from build123d import *

# Parameters (mm, degrees)
F0_W     = 3
F0_H     = 20
F0_W_2   = 2
F0_H_2   = 4
F1_DEPTH = 3
F3_W     = 4
F3_H     = 2
F4_DEPTH = 3


with BuildPart() as f1:
    # F0 (on Top) → F1 (new body)
    with BuildSketch(Plane.XY):
        Polygon((-25, 0), (-30, 0), (-30, -50), (0, 0), align=None)
        with Locations((-23.5, -20)):
            Rectangle(F0_W, F0_H, mode=Mode.SUBTRACT)
        Polygon((0, 0), (-30, -50), (-30, -100), (0, -100), (30, -100), (30, -50), (30, 0), align=None)
        with Locations((-23.5, -80)):
            Rectangle(F0_W, F0_H, mode=Mode.SUBTRACT)
        Polygon((12.9807621135, -87.5470053838), (0, -80.0525588833), (-0.0096189432, -80.0470053838), (-13, -87.5470053838), (-13, -81.7735026919), (-0.0096189432, -74.2735026919), (12.9807621135, -81.7735026919), align=None, mode=Mode.SUBTRACT)
        Polygon((-13, -70), (-0.0096189432, -62.5), (12.9807621135, -70), (12.9807621135, -75.7735026919), (-0.0096189432, -68.2735026919), (-13, -75.7735026919), align=None, mode=Mode.SUBTRACT)
        with Locations((23.5, -80)):
            Rectangle(F0_W, F0_H, mode=Mode.SUBTRACT)
        with Locations((28, -52)):
            Rectangle(F0_W_2, F0_H_2, mode=Mode.SUBTRACT)
        Polygon((-12.9903810568, -39.2735026919), (0, -31.7735026919), (12.9903810568, -39.2735026919), (12.9903810568, -45.0470053838), (0, -37.5470053838), (-12.9903810568, -45.0470053838), align=None, mode=Mode.SUBTRACT)
        Polygon((-12.9903810568, -27.5), (0, -20), (12.9903810568, -27.5), (12.9903810568, -33.2735026919), (0, -25.7735026919), (-12.9903810568, -33.2735026919), align=None, mode=Mode.SUBTRACT)
        with Locations((23.5, -20)):
            Rectangle(F0_W, F0_H, mode=Mode.SUBTRACT)
    extrude(amount=F1_DEPTH)

    # F3 (on offset) → F4 (cut, through all)
    with BuildSketch(Plane.YZ.offset(30)):
        with Locations((-52, 1.5)):
            Rectangle(F3_W, F3_H)
    extrude(amount=-F4_DEPTH, mode=Mode.SUBTRACT)


solid = f1.part
Check sheet for the modelled part. Datum: model origin and axes. Units: mm. Coordinates: 2 decimals unless noted, no trailing zeros. Write each loop counter-clockwise with the first axis right and the second up, starting at its lowest first coordinate (ties: lowest second). Pieces come first, ordered by that corner, then holes.
Item 1: Cross-section at A-A on y = -89. Record the boundary of the cut face in (x, z), then the cut area to 3 significant figures.
Numbers:
outline: (-30, 0) - (-25, 0) - (-25, 3) - (-30, 3) - close; (-22, 0) - (22, 0) - (22, 3) - (-22, 3) - close; (25, 0) - (30, 0) - (30, 3) - (25, 3) - close
area: 162 mm2
Item 2: Cross-section at D-D on y = -36.5. Record the boundary of the cut face in (x, z), then the cut area to 3 significant figures.
Numbers:
outline: (-30, 0) - (-8.19, 0) - (-8.19, 3) - (-30, 3) - close; (8.19, 0) - (30, 0) - (30, 3) - (8.19, 3) - close
area: 131 mm2
Item 3: Cross-section at B-B on y = -72. Record the boundary of the cut face in (x, z).
Numbers:
outline: (-30, 0) - (-25, 0) - (-25, 3) - (-30, 3) - close; (-22, 0) - (-13, 0) - (-13, 3) - (-22, 3) - close; (-6.46, 0) - (6.44, 0) - (6.44, 3) - (-6.46, 3) - close; (12.98, 0) - (22, 0) - (22, 3) - (12.98, 3) - close; (25, 0) - (30, 0) - (30, 3) - (25, 3) - close
Item 4: Scan lines: probe 1 along X at (y, z) = (-18.5, 2); probe 2 along Y at (x, z) = (24.5, 1.65); probe 3 along Y at (x, z) = (-12, 0.3). Record each from-to range of solid material in increasing order.
Numbers:
probe 1: x = -30 to -25, -22 to 22, 25 to 30
probe 2: y = -100 to -90, -70 to -30, -10 to 0
probe 3: y = -100 to -86.97, -81.2 to -75.2, -69.42 to -44.48, -38.7 to -32.7, -26.93 to 0
Item 5: Mould release check, pull along Y, two halves, no side actions. Record for faces 1 (the face through (30, -50.7, 2.8)), 2 (the face through (-6.59, -35.58, 1.48)): released by +Y, released by -Y, zero draft, split by the parting line, or undercut.
Numbers:
face 1: zero draft
face 2: undercut
Item 6: Cross-section at C-C on x = -11. Record the boundary of the cut face in (y, z), then the cut area to 3 significant figures.
Numbers:
outline: (-100, 0) - (-86.39, 0) - (-86.39, 3) - (-100, 3) - close; (-80.62, 0) - (-74.62, 0) - (-74.62, 3) - (-80.62, 3) - close; (-68.85, 0) - (-43.9, 0) - (-43.9, 3) - (-68.85, 3) - close; (-38.12, 0) - (-32.12, 0) - (-32.12, 3) - (-38.12, 3) - close; (-26.35, 0) - (0, 0) - (0, 3) - (-26.35, 3) - close
area: 231 mm2
